Source: CAD feature listing. Evaluate the final solid. Frame: model axes, mm. A direction names the side the tool comes from. Give positions to 0.01 mm unless a question says otherwise; leave off trailing zeros. Order: outer loops, then holes, each group sorted by start corner. A loop starts at its lowest first (then second) coordinate and runs counter-clockwise, first axis right, second up. Notation, with made-up numbers: (27, 85.5) - (70, 85.5) arc R13 ccw to (70, 102.5) - close; hole circle Ø5 at (34, 5). An arc over 180 degrees is marked (long way). Answer as CSV lines item,"result".
Autodesk Inventor part; units mm, degrees
ref_plane "YZ Plane" through (0, 0, 0) normal (1, 0, 0) x (0, 1, 0)
ref_plane "XZ Plane" through (0, 0, 0) normal (0, 1, 0) x (-1, 0, 0)
ref_plane "XY Plane" through (0, 0, 0) normal (0, 0, 1) x (1, 0, 0)
sketch "Sketch1" plane through (0, 0, 0) normal (0, 0, 1) x (1, 0, 0)
  line L0 (-48, 48) -> (48, 48)
  line L1 (48, 48) -> (48, -48)
  line L2 (48, -48) -> (-48, -48)
  line L3 (-48, -48) -> (-48, 48)
  line L4 (38, 38) -> (-38, 38)
  line L5 (-38, 38) -> (-38, -38)
  line L6 (-38, -38) -> (38, -38)
  line L7 (38, -38) -> (38, 38)
  line L8 (0, 152.7233) -> (0, -72.1628) construction
  line L9 (-77.8847, 0) -> (88.8171, 0) construction
  line L10 (-48, 43) -> (48, 43) construction
  line L11 (-43, 48) -> (-43, -48) construction
  line L12 (-48, -43) -> (48, -43) construction
  circle A0 centre (-43, 25) radius 2.25
  circle A1 centre (-43, -25) radius 2.25
  circle A2 centre (-43, -43) radius 2.25
  circle A3 centre (-43, 43) radius 2.25
  line L13 (-48, 30) -> (48, 30) construction
  line L14 (-48, -30) -> (48, -30) construction
  line L15 (-50, 31) -> (-36, 31)
  line L16 (-36, 31) -> (-36, -31)
  line L17 (-36, -31) -> (-50, -31)
  line L18 (-50, -31) -> (-50, 31)
  point P0 (0, 0)
  point P1 (0, 48)
  point P2 (48, 0)
  dimension "d0" = 96
  dimension "d1" = 96
  dimension "d2" = 10
  dimension "d5" = 5
  dimension "d11" = 5
  dimension "d14" = 5
  dimension "d31" = 4.5
  dimension "d32" = 4.5
  dimension "d61" = 4.5
  dimension "d62" = 4.5
  dimension "d65" = 30
  dimension "d66" = 30
  dimension "d67" = 5
  dimension "d68" = 5
  dimension "d74" = 1
  dimension "d75" = 1
  dimension "d76" = 2
  dimension "d77" = 2
extrude "Extrusion1" add sketch "Sketch1" against normal blind 1.5 contours L0 L1 L2 L3 L17 L5 L6 L7 L4 L15 | L15 L5 L17 L3 | A0 | A1 | A2 | A3
extrude "Extrusion2" cut sketch "Sketch1" against normal blind 10 contours A2 | A3
mirror "Mirror5" about plane through (0, 0, 0) normal (1, 0, 0) of "Extrusion2"
extrude "Extrusion5" cut sketch "Sketch1" against normal blind 10 contours A0 | A1
pattern_circular "Circular Pattern1" count 4 over 360 about axis through (0, 0, -10) along (0, 0, 1) of "Extrusion5"
sketch "Sketch3" plane through (0, 0, 0) normal (0, 0, 1) x (1, 0, 0)
  circle A0 centre (25, 43) radius 2.25
  circle A1 centre (-25, 43) radius 2.25
  circle A2 centre (43, -25) radius 2.25
  circle A3 centre (43, 25) radius 2.25
  circle A4 centre (-25, -43) radius 2.25
  circle A5 centre (25, -43) radius 2.25
  circle A6 centre (-43, 25) radius 2.25
  circle A7 centre (-43, -25) radius 2.25
  circle A8 centre (43, -43) radius 2.25
  circle A9 centre (43, 43) radius 2.25
  circle A10 centre (-43, -43) radius 2.25
  circle A11 centre (-43, 43) radius 2.25
  line L0 (-38, -38) -> (-38, 38)
  line L1 (-38, 38) -> (38, 38)
  line L2 (38, 38) -> (38, -38)
  line L3 (38, -38) -> (-38, -38)
  line L4 (-48, 48) -> (48, 48)
  line L5 (-48, -48) -> (-48, 48)
  line L6 (48, -48) -> (-48, -48)
  line L7 (48, 48) -> (48, -48)
  circle A12 centre (0, 0) radius 7.5
  circle A13 centre (0, 0) radius 12.5
  line L8 (-35.5251, 40.4749) -> (40.4749, -35.5251)
  line L9 (40.4749, -35.5251) -> (35.5251, -40.4749)
  line L10 (35.5251, -40.4749) -> (-40.4749, 35.5251)
  line L11 (-40.4749, 35.5251) -> (-35.5251, 40.4749)
  line L12 (-38, 38) -> (38, -38) construction
  line L13 (2.4749, 2.4749) -> (-2.4749, -2.4749) construction
  dimension "d80" = 15
  dimension "d81" = 5
  dimension "d82" = 7
extrude "Extrusion7" add sketch "Sketch3" against normal blind 1 contours L10 A12 A13 | A13 L8 A12 L10 | L10 A12 L8 A13 | A13 L8 A12
extrude "Extrusion8" add sketch "Sketch3" against normal blind 1 contours L10 L11 L0 | L0 L1 L8 A13 L10 | L10 A13 L8 L2 L3 | L3 L9 L10 | L11 L8 L1 | A13 L8 A12 L10 | L2 L8 L9 | L10 A12 L8 A13 | A12 L8 L10
mirror "Mirror6" about plane through (0, 0, 0) normal (1, 0, 0) of "Extrusion8"
extrude "Extrusion9" cut sketch "Sketch3" against normal blind 1 contours L10 A12 | A12 L8 L10 | A12 L8
sketch "Sketch4" plane through (0, 0, -1.5) normal (0, 0, -1) x (-1, 0, 0)
  line L0 (48, -48) -> (48, 48)
  line L1 (38, -33.0503) -> (38, 33.0503)
  line L2 (48, -17.5) -> (38, -17.5)
  line L3 (38, -17.5) -> (38, 17.5)
  line L4 (38, 17.5) -> (48, 17.5)
  line L5 (48, 17.5) -> (48, -17.5)
  point P0 (0, 0)
  point P1 (38, 0)
  point P2 (38, 0)
  dimension "d89" = 35
extrude "Extrusion10" add sketch "Sketch4" along normal blind 5
pattern_circular "Circular Pattern2" count 4 over 360 about axis through (0, 0, -10) along (0, 0, 1) of "Extrusion10"
equation "\"d31\" = screw"
equation "\"d32\" = screw"
equation "\"d61\" = screw"
equation "\"d62\" = screw"
properties part number "Base" material "PC/ABS Plastic"
(1) Cut plane B-B (z = -4.5). Return loops of the section in (x, y).
Completed:
outline,"(-48, -17.5) - (-38, -17.5) - (-38, 17.5) - (-48, 17.5) - close; (-17.5, -48) - (17.5, -48) - (17.5, -38) - (-17.5, -38) - close; (-17.5, 38) - (17.5, 38) - (17.5, 48) - (-17.5, 48) - close; (38, -17.5) - (48, -17.5) - (48, 17.5) - (38, 17.5) - close"
(2) Contact query for flat-ended pins moving along their axis: pin 1 (9 mm diameter, centred on x = 0, y = 0, fed in from +Z); pin 2 (24.5 mm diameter, centred on x = -30.5, y = -28.5, fed in from -Z); pin 3 (5 mm diameter, centred on x = -43, y = -25, fed in from +Z); pin 4 (8 mm diameter, centred on x = 10, y = -6.5, fed in from -Z). Output: stop coordinate, or through.
Completed:
pin 1,"through"
pin 2,"z = -1.5"
pin 3,"z = 0"
pin 4,"z = -1"
(3) Mould query, pull axis X, two halves, no side actions, for faces 1 (the flat face through (17.5, -43, -4)), 2 (the cylindrical face through (43.29, -45.23, -0.74)), 3 (the flat face through (39, -36, -1.5)). Classes: released by +X, released by -X, zero draft, split by the parting line, or undercut.
Completed:
face 1,"released by +X"
face 2,"undercut"
face 3,"zero draft"
(4) Cut plane C-C (x = 0). Return loops of the section in (y, z).
Completed:
outline,"(-48, -6.5) - (-38, -6.5) - (-38, 0) - (-48, 0) - close; (-12.5, -1) - (-7.5, -1) - (-7.5, 0) - (-12.5, 0) - close; (7.5, -1) - (12.5, -1) - (12.5, 0) - (7.5, 0) - close; (38, -6.5) - (48, -6.5) - (48, 0) - (38, 0) - close"
(5) Ray query, line 1 (Y direction, x = 43, z = -0.6); line 2 (X direction, y = 0, z = -0.5); line 3 (X direction, y = -13.5, z = -4). Return the intervals inside material, ascending. Write a range as from..to.
Completed:
line 1,"-48..-45.25, -40.75..-27.25, -22.75..22.75, 27.25..40.75, 45.25..48"
line 2,"-48..-38, -12.5..-7.5, 7.5..12.5, 38..48"
line 3,"-48..-38, 38..48"
(6) Cut plane A-A (y = -43). Return loops of the section in (x, z), then the cut area to 3 significant figures.
Completed:
outline,"(-48, -1.5) - (-45.25, -1.5) - (-45.25, 0) - (-48, 0) - close; (-40.75, -1.5) - (-27.25, -1.5) - (-27.25, 0) - (-40.75, 0) - close; (-22.75, -1.5) - (-17.5, -1.5) - (-17.5, -6.5) - (17.5, -6.5) - (17.5, -1.5) - (22.75, -1.5) - (22.75, 0) - (-22.75, 0) - close; (27.25, -1.5) - (40.75, -1.5) - (40.75, 0) - (27.25, 0) - close; (45.25, -1.5) - (48, -1.5) - (48, 0) - (45.25, 0) - close"
area,"292 mm²"
(7) Access query for faces 4 (the flat face through (19.34, 24.29, -0.49)), 5 (the flat face through (17.5, 43, -4)), 6 (the flat face through (36, 40, -1.5)), 7 (the flat face through (-17.5, -43, -4)). Directions: +Z, -Z, +X, -X, +Y, -Y. A direction counts if a zero-diameter tool reaches every point of the face in a straight line with its end or side. Return the directions, or none.
Completed:
face 4,"+Z, -Z"
face 5,"-Z, +X, +Y, -Y"
face 6,"-Z, +X, +Y"
face 7,"-Z, -X, +Y, -Y"
